For this review, take the finished solid that the model builds, in its own axes (mm). A direction names the side the tool comes from. Coordinates: 2 decimals unless noted, no trailing zeros. Write each loop counter-clockwise with the first axis right and the second up, starting at its lowest first coordinate (ties: lowest second). Pieces come first, ordered by that corner, then holes. Notation, with made-up numbers: (-16.5, 89) -> (32.5, 89) arc R34 cw to (32.5, 126) -> close; hole circle Ø4 at (71.5, 87). An arc over 180 degrees is marked (long way). One line per item, written item: value. Start each with the question number.
1) Add section D-D (x = -24). State the section outline as (y, z) points, and give its area (3 significant figures).
2) Machinability: for faces 1 (the flat face through (-26, -19, -5.375)), 2 (the flat face through (16.6, -15.7, -5.375)), 3 (the flat face through (-3, 0, -6)), which of the approach directions +Z, -Z, +X, -X, +Y, -Y give a long, thin tool a straight path to every point of the face, cutting with its end or side? Answer none if there is none.
3) Add section A-A (x = -5). State the section outline as (y, z) points, and give its area (3 significant figures).
4) Add section B-B (y = -11). State the section outline as (x, z) points.
5) For probe 1 along Z at (x, y) = (-10, -12.5); probe 2 along X at (y, z) = (-10.5, -11); probe 3 along Y at (x, z) = (-11.5, 14), list the stretches that pass through material, from the lowest coordinate up. Write a range as from..to.
6) Add section C-C (z = 12.5). State the section outline as (x, y) points.
7) For pin 1 Ø12 at (y, z) = (-19, 0) entering from +X; pin 2 Ø5 at (x, y) = (19.5, -17) entering from +Z; pin 3 Ø4 at (y, z) = (-6, -6.5) entering from +X, all flat-tipped, find the tip position at first contact; note any pin that passes through.
from build123d import *

# Parameters (mm, degrees)
F0_W     = 76.2
F0_H     = 44.45
F1_DEPTH = 25.4
F2_W     = 25.4
F2_H     = 31.75
F3_DEPTH = 25.401
F5_DEPTH = 50.801
F7_DEPTH = 12.701
F9_DEPTH = 12.701


with BuildPart() as f1:
    # F0 (on Front) → F1 (new body)
    with BuildSketch(Plane.XZ):
        with Locations((-3.0154539272, 4.1499344332)):
            Rectangle(F0_W, F0_H)
    extrude(amount=F1_DEPTH)

    # F2 (on face) → F3 (cut, through all)
    with BuildSketch(Plane.XZ.offset(25.4)):
        with Locations((-28.4154539272, 10.4999344332)):
            Rectangle(F2_W, F2_H)
        with Locations((22.3845460728, 10.4999344332)):
            Rectangle(F2_W, F2_H)
    extrude(amount=-F3_DEPTH, mode=Mode.SUBTRACT)

    # F4 (on face) → F5 (cut, through all)
    with BuildSketch(Plane.YZ.offset(9.6845460728)):
        with BuildLine():
            ThreePointArc((-12.7, 20.0249344332), (-17.1901280646, 18.1650624897), (-19.05, 13.6749344217))
            Line((-19.05, 13.6749344332), (-6.35, 13.6749344332))
            ThreePointArc((-6.35, 13.6749344332), (-8.2098719395, 18.1650624937), (-12.7, 20.0249344332))
        make_face()
        with BuildLine():
            Line((-6.35, 13.6749344332), (-19.05, 13.6749344332))
            ThreePointArc((-19.05, 13.6749344217), (-17.1901280565, 9.1848063686), (-12.7, 7.3249344332))
            ThreePointArc((-12.7, 7.3249344332), (-8.2098719395, 9.1848063726), (-6.35, 13.6749344332))
        make_face()
        with BuildLine():
            Line((-6.35, 26.3749344332), (-6.35, 24.6734570612))
            ThreePointArc((-6.35, 24.6734570612), (-3.7197438789, 22.6551905542), (-1.7014773719, 20.0249344332))
            Line((-1.7014773719, 20.0249344332), (0, 20.0249344332))
            Line((0, 20.0249344332), (0, 26.3749344332))
            Line((0, 26.3749344332), (-6.35, 26.3749344332))
        make_face()
        with BuildLine():
            Line((-25.4, 26.3749344332), (-25.4, 20.0249344332))
            Line((-25.4, 20.0249344332), (-23.6985226281, 20.0249344332))
            ThreePointArc((-23.6985226281, 20.0249344332), (-21.6802561211, 22.6551905542), (-19.05, 24.6734570612))
            Line((-19.05, 24.6734570612), (-19.05, 26.3749344332))
            Line((-19.05, 26.3749344332), (-25.4, 26.3749344332))
        make_face()
        with BuildLine():
            Line((-19.05, 26.3749344332), (-19.05, 24.6734570612))
            ThreePointArc((-19.05, 24.6734570612), (-15.9870018728, 25.942192427), (-12.7, 26.3749344332))
            Line((-12.7, 26.3749344332), (-19.05, 26.3749344332))
        make_face()
        with BuildLine():
            Line((-6.35, 26.3749344332), (-12.7, 26.3749344332))
            ThreePointArc((-12.7, 26.3749344332), (-9.4129981272, 25.942192427), (-6.35, 24.6734570612))
            Line((-6.35, 24.6734570612), (-6.35, 26.3749344332))
        make_face()
        with BuildLine():
            Line((-23.6985226281, 20.0249344332), (-25.4, 20.0249344332))
            Line((-25.4, 20.0249344332), (-25.4, 13.6749344332))
            ThreePointArc((-25.4, 13.6749344332), (-24.9672579939, 16.961936306), (-23.6985226281, 20.0249344332))
        make_face()
        with BuildLine():
            ThreePointArc((-1.7014773719, 20.0249344332), (-0.4327420061, 16.961936306), (0, 13.6749344332))
            Line((0, 13.6749344332), (0, 20.0249344332))
            Line((0, 20.0249344332), (-1.7014773719, 20.0249344332))
        make_face()
    extrude(amount=-F5_DEPTH, mode=Mode.SUBTRACT)

    # F6 (on face) → F7 (cut, through all)
    with BuildSketch(Plane.XY.offset(-5.3750655668)):
        with BuildLine():
            ThreePointArc((-22.0654539272, -12.7), (-23.9253258667, -8.2098719395), (-28.4154539272, -6.35))
            Line((-28.4154539272, -6.35), (-28.4154539272, -19.05))
            ThreePointArc((-28.4154539272, -19.05), (-23.9253258667, -17.1901280605), (-22.0654539272, -12.7))
        make_face()
        with BuildLine():
            Line((-28.4154539272, -19.05), (-28.4154539272, -6.35))
            ThreePointArc((-28.4154539272, -6.35), (-32.9055819878, -8.2098719395), (-34.7654539272, -12.7))
            ThreePointArc((-34.7654539272, -12.7), (-32.9055819878, -17.1901280605), (-28.4154539272, -19.05))
        make_face()
        with BuildLine():
            Line((-34.7654539272, -1.7014773719), (-34.7654539272, 0))
            Line((-34.7654539272, 0), (-41.1154539272, 0))
            Line((-41.1154539272, 0), (-41.1154539272, -6.35))
            Line((-41.1154539272, -6.35), (-39.4139765553, -6.35))
            ThreePointArc((-39.4139765553, -6.35), (-37.3957100483, -3.7197438789), (-34.7654539272, -1.7014773719))
        make_face()
        with BuildLine():
            ThreePointArc((-41.1154539272, -12.7), (-40.6827119211, -9.4129981272), (-39.4139765553, -6.35))
            Line((-39.4139765553, -6.35), (-41.1154539272, -6.35))
            Line((-41.1154539272, -6.35), (-41.1154539272, -12.7))
        make_face()
        with BuildLine():
            Line((-28.4154539272, 0), (-34.7654539272, 0))
            Line((-34.7654539272, 0), (-34.7654539272, -1.7014773719))
            ThreePointArc((-34.7654539272, -1.7014773719), (-31.7024558, -0.4327420061), (-28.4154539272, 0))
        make_face()
        with BuildLine():
            ThreePointArc((-39.4139765553, -19.05), (-40.6827119211, -15.9870018728), (-41.1154539272, -12.7))
            Line((-41.1154539272, -12.7), (-41.1154539272, -19.05))
            Line((-41.1154539272, -19.05), (-39.4139765553, -19.05))
        make_face()
        with BuildLine():
            ThreePointArc((-34.7654539272, -23.6985226281), (-37.3957100483, -21.6802561211), (-39.4139765553, -19.05))
            Line((-39.4139765553, -19.05), (-41.1154539272, -19.05))
            Line((-41.1154539272, -19.05), (-41.1154539272, -25.4))
            Line((-41.1154539272, -25.4), (-34.7654539272, -25.4))
            Line((-34.7654539272, -25.4), (-34.7654539272, -23.6985226281))
        make_face()
        with BuildLine():
            Line((-34.7654539272, -25.4), (-28.4154539272, -25.4))
            ThreePointArc((-28.4154539272, -25.4), (-31.7024558, -24.9672579939), (-34.7654539272, -23.6985226281))
            Line((-34.7654539272, -23.6985226281), (-34.7654539272, -25.4))
        make_face()
    extrude(amount=-F7_DEPTH, mode=Mode.SUBTRACT)

    # F8 (on face) → F9 (cut, through all)
    with BuildSketch(Plane.XY.offset(-5.3750655668)):
        with BuildLine():
            ThreePointArc((28.7345460728, -12.7), (26.8746741333, -8.2098719395), (22.3845460728, -6.35))
            Line((22.3845460728, -6.35), (22.3845460728, -19.05))
            ThreePointArc((22.3845460728, -19.05), (26.8746741333, -17.1901280605), (28.7345460728, -12.7))
        make_face()
        with BuildLine():
            ThreePointArc((22.3845460728, -6.35), (17.8944180122, -8.2098719395), (16.0345460728, -12.7))
            ThreePointArc((16.0345460728, -12.7), (17.8944180122, -17.1901280605), (22.3845460728, -19.05))
            Line((22.3845460728, -19.05), (22.3845460728, -6.35))
        make_face()
        with BuildLine():
            ThreePointArc((28.7345460728, -23.6985226281), (25.6715479456, -24.9672579939), (22.3845460728, -25.4))
            Line((22.3845460728, -25.4), (28.7345460728, -25.4))
            Line((28.7345460728, -25.4), (28.7345460728, -23.6985226281))
        make_face()
        with BuildLine():
            ThreePointArc((33.3830687008, -19.05), (31.3648021939, -21.6802561211), (28.7345460728, -23.6985226281))
            Line((28.7345460728, -23.6985226281), (28.7345460728, -25.4))
            Line((28.7345460728, -25.4), (35.0845460728, -25.4))
            Line((35.0845460728, -25.4), (35.0845460728, -19.05))
            Line((35.0845460728, -19.05), (33.3830687008, -19.05))
        make_face()
        with BuildLine():
            Line((35.0845460728, -19.05), (35.0845460728, -12.7))
            ThreePointArc((35.0845460728, -12.7), (34.6518040667, -15.9870018728), (33.3830687008, -19.05))
            Line((33.3830687008, -19.05), (35.0845460728, -19.05))
        make_face()
        with BuildLine():
            Line((35.0845460728, -6.35), (33.3830687008, -6.35))
            ThreePointArc((33.3830687008, -6.35), (34.6518040667, -9.4129981272), (35.0845460728, -12.7))
            Line((35.0845460728, -12.7), (35.0845460728, -6.35))
        make_face()
        with BuildLine():
            Line((28.7345460728, 0), (28.7345460728, -1.7014773719))
            ThreePointArc((28.7345460728, -1.7014773719), (31.3648021939, -3.7197438789), (33.3830687008, -6.35))
            Line((33.3830687008, -6.35), (35.0845460728, -6.35))
            Line((35.0845460728, -6.35), (35.0845460728, 0))
            Line((35.0845460728, 0), (28.7345460728, 0))
        make_face()
        with BuildLine():
            Line((28.7345460728, 0), (22.3845460728, 0))
            ThreePointArc((22.3845460728, 0), (25.6715479456, -0.4327420061), (28.7345460728, -1.7014773719))
            Line((28.7345460728, -1.7014773719), (28.7345460728, 0))
        make_face()
    extrude(amount=-F9_DEPTH, mode=Mode.SUBTRACT)


solid = f1.part
Numbers:
1. outline: (-25.4, -18.08) -> (-17.26, -18.08) -> (-17.26, -5.38) -> (-25.4, -5.38) -> close; (-8.14, -18.08) -> (0, -18.08) -> (0, -5.38) -> (-8.14, -5.38) -> close
1. area: 207 mm²
2. face 1: +Z, -X, +Y, -Y
2. face 2: +Z, +X, +Y, -Y
2. face 3: +Z, -Z, +X, -X, +Y
3. outline: (-25.4, -18.08) -> (0, -18.08) -> (0, 13.67) arc R12.7 ccw to (-25.4, 13.67) -> close; hole circle Ø12.7 at (-12.7, 13.67)
3. area: 933 mm²
4. outline: (-41, -18.08) -> (-34.53, -18.08) -> (-34.53, -5.38) -> (-41, -5.38) -> close; (-22.3, -18.08) -> (16.27, -18.08) -> (16.27, -5.38) -> (9.68, -5.38) -> (9.68, 7.56) -> (-15.72, 7.56) -> (-15.72, -5.38) -> (-22.3, -5.38) -> close; (-15.72, 19.79) -> (9.68, 19.79) -> (9.68, 26.26) -> (-15.72, 26.26) -> close; (28.5, -18.08) -> (34.97, -18.08) -> (34.97, -5.38) -> (28.5, -5.38) -> close
5. probe 1: -18.08..7.33, 20.02..26.37
5. probe 2: -40.92..-34.37, -22.46..16.43, 28.34..34.89
5. probe 3: -25.4..-19.04, -6.36..0
6. outline: (-15.72, -25.4) -> (9.68, -25.4) -> (9.68, -18.94) -> (-15.72, -18.94) -> close; (-15.72, -6.46) -> (9.68, -6.46) -> (9.68, 0) -> (-15.72, 0) -> close
7. pin 1: x = 34.55
7. pin 2: z = -5.38
7. pin 3: x = 34.18
